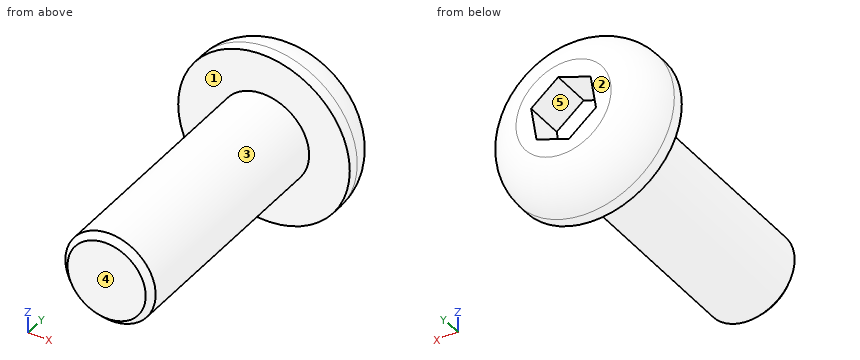
Autodesk Inventor part; units mm, degrees
ref_plane "YZ Plane" through (0, 0, 0) normal (1, 0, 0) x (0, 1, 0)
ref_plane "XZ Plane" through (0, 0, 0) normal (0, 1, 0) x (-1, 0, 0)
ref_plane "XY Plane" through (0, 0, 0) normal (0, 0, 1) x (1, 0, 0)
sketch "Sketch1" plane through (0, 0, 0) normal (0, 0, 1) x (1, 0, 0)
  line L0 (-10.627, -30.5907) -> (-13.477, -30.5907)
  line L1 (-10.627, -30.5907) -> (-10.627, -38.5907)
  line L2 (-10.627, -38.5907) -> (-12.127, -38.5907)
  line L3 (-12.127, -38.5907) -> (-12.127, -30.5907)
  line L4 (-10.627, -30.5907) -> (-10.627, -26.5988)
  line L5 (-13.477, -30.5907) -> (-13.477, -30.2107)
  line L6 (-13.477, -30.2107) -> (-13.477, -28.9407)
  line L7 (-13.477, -28.9407) -> (-10.627, -28.9407)
  point P0 (0, 0)
  dimension "d0" = 2.85
  dimension "d2" = 8
  dimension "d3" = 1.5
  dimension "d18" = 0.38
  dimension "d19" = 1.65
revolve "Revolution1" add sketch "Sketch1" angle 360 about axis through (-10.627, -30.5907, 0) along (0, -1, 0)
chamfer "Chamfer2" distance 0.2 angle 45 1 edges at (-9.127, -38.5907, 0)
fillet "Empalme2" radius 1.27 1 edges at (-7.777, -28.9407, 0)
sketch "Boceto2" plane through (-10.627, -28.9407, 0) normal (0, 1, 0) x (1, 0, 0)
  line L0 (0.8985, 0.7252) -> (1.0773, -0.4156)
  line L1 (1.0773, -0.4156) -> (0.1788, -1.1408)
  line L2 (0.1788, -1.1408) -> (-0.8985, -0.7252)
  line L3 (-0.8985, -0.7252) -> (-1.0773, 0.4156)
  line L4 (-1.0773, 0.4156) -> (-0.1788, 1.1408)
  line L5 (-0.1788, 1.1408) -> (0.8985, 0.7252)
  point P0 (10.627, 0)
  point P1 (0, 0)
  dimension "d21" = 2
extrude "Extrusión1" cut sketch "Boceto2" against normal blind 1.3
thread "Rosca2"
properties part number "Tornillo Allen cabeeza botón M3x8mm"
Geometry check sheet. Reference: the model listing, model coordinates, mm. Face numbers are marked on the shaded views. A direction names the side the tool comes from. Round coordinates to 2 decimals unless told otherwise and drop trailing zeros. Loops run counter-clockwise (first coordinate to the right, second up) from the corner with the lowest first, then second, coordinate; pieces in that order, holes last.
Item 1: Cross-section at B-B on z = 0. Record the boundary of the cut face in (x, y).
Item 2: Gauge pin test, flat ends, axial feed: pin 1 (1.5 mm diameter, centred on y = -32.5, z = 1, fed in from +X); pin 2 (1.5 mm diameter, centred on y = -30.5, z = 2, fed in from +X); pin 3 (1.5 mm diameter, centred on x = -10, y = -34.5, fed in from +Z). Record the tip position at first contact, or that the pin passes through.
Item 3: Mould release check, pull along Y, two halves, no side actions. Record for the marked faces 1, 2 and 3: pulls with the +Y half, pulls with the -Y half, needs draft (parallel to the pull), parting line crosses it, or undercut.
Item 4: Thickness scan on line 1 (Z direction, x = -11.6, y = -32.25); line 2 (Y direction, x = -10.6, z = -1.6); line 3 (Y direction, x = -10.3, z = -0.1). Record the ranges inside material, lowest first.
Item 5: Cross-section at A-A on y = -36.75. Record the boundary of the cut face in (x, z), then the cut area to 3 significant figures.
Item 6: Access from +Z, -Z, +X, -X, +Y, -Y to the whole of each face (thin tool, end or side, straight path). Record for the marked faces 4 and 5.
Answer sheet:
1. outline: (-13.48, -30.59) - (-12.13, -30.59) - (-12.13, -38.39) - (-11.93, -38.59) - (-9.33, -38.59) - (-9.13, -38.39) - (-9.13, -30.59) - (-7.78, -30.59) - (-7.78, -30.21) arc R1.27 ccw to (-9.05, -28.94) - (-9.61, -28.94) - (-9.61, -30.24) - (-11.64, -30.24) - (-11.64, -28.94) - (-12.21, -28.94) arc R1.27 ccw to (-13.48, -30.21) - close
2. pin 1: stops at x = -9.15
2. pin 2: stops at x = -8.07
2. pin 3: stops at z = 1.5
3. face 1: pulls with the -Y half
3. face 2: pulls with the +Y half
3. face 3: needs draft
4. line 1: z = -1.14 to 1.14
4. line 2: y = -30.59 to -28.94
4. line 3: y = -38.59 to -30.24
5. outline: circle Ø3 at (-10.63, 0)
5. area: 7.07 mm2
6. face 4: +Z, -Z, +X, -X, -Y
6. face 5: +Y
